The model under review builds one solid part; all positions refer to its coordinate system, in mm. Coordinates: 2 decimals unless noted, no trailing zeros. Loops run counter-clockwise (first coordinate to the right, second up) from the corner with the lowest first, then second, coordinate; pieces in that order, holes last. Notation, with made-up numbers: M -33,-40 L 12,-40 A21 ccw 12,-18 Z; hole C 16,-23 d4. An arc over 180 degrees is marked long. Return JSON: item names as keys, results as strings.
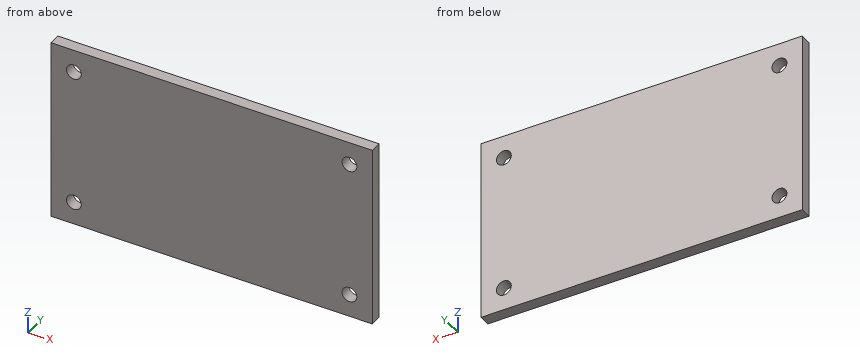
```python
from build123d import *

# Parameters (mm, degrees)
SKETCH1_W                = 177.8
SKETCH1_H                = 101.6
BOSS_EXTRUDE1_DEPTH      = 6.35
P_0_323_DIAMETER_HOLE1_D = 8.2042


with BuildPart() as part:
    # Sketch1 → Boss-Extrude1 (new body)
    with BuildSketch(Plane(origin=(0, 0, 0), x_dir=(1, 0, 0), z_dir=(0, 1, 0))):
        Rectangle(SKETCH1_W, SKETCH1_H)
    extrude(amount=-BOSS_EXTRUDE1_DEPTH)

    # P (0.323) Diameter Hole1 (through all)
    with Locations(Plane(origin=(0, 0, 0), x_dir=(1, 0, 0), z_dir=(0, 1, 0))):
        with Locations((-76.2, 38.1), (-76.2, -38.1), (76.2, -38.1), (76.2, 38.1)):
            Hole(P_0_323_DIAMETER_HOLE1_D / 2)


solid = part.part
```
1. Insertion check: pin 1 Ø10.5 at (x, z) = (76.2, -38.1) entering from -Y. The pin has a flat end and moves straight along its axis. Give the tip position at first contact, or say it passes through.
Check values:
{"pin 1": "y = -6.35"}
2. Add section B-B on x = -76.2. Give the boundary of the cut face in (y, z).
Check values:
{"outline": "M -6.35,-50.8 L 0,-50.8 L 0,-42.2 L -6.35,-42.2 Z; M -6.35,-34 L 0,-34 L 0,34 L -6.35,34 Z; M -6.35,42.2 L 0,42.2 L 0,50.8 L -6.35,50.8 Z"}
3. Add section A-A on z = -38.1. Give the boundary of the cut face in (x, y), plus the area to 3 significant figures.
Check values:
{"outline": "M -88.9,-6.35 L -80.3,-6.35 L -80.3,0 L -88.9,0 Z; M -72.1,-6.35 L 72.1,-6.35 L 72.1,0 L -72.1,0 Z; M 80.3,-6.35 L 88.9,-6.35 L 88.9,0 L 80.3,0 Z", "area": "1,020 mm²"}
4. To check wall thickness, follow line 1 (Z direction, x = -76.2, y = -3); line 2 (X direction, y = -4, z = -38.1); line 3 (X direction, y = -4.5, z = -39). State the ranges of each line that lie inside material, in increasing order.
Check values:
{"line 1": "-50.8 to -42.2, -34 to 34, 42.2 to 50.8", "line 2": "-88.9 to -80.3, -72.1 to 72.1, 80.3 to 88.9", "line 3": "-88.9 to -80.2, -72.2 to 72.2, 80.2 to 88.9"}
